Design review of the part built by this model. Coordinates are the model's own, in mm. Give positions to 0.01 mm unless a question says otherwise; leave off trailing zeros. Answer as a JSON object with one key per item and string values.
Autodesk Inventor part; units mm, degrees
ref_plane "Start Plane" through (0, 0, 0) normal (0, 0, 1) x (1, 0, 0)
ref_plane "End Plane" through (0, 0, 400) normal (0, 0, 1) x (1, 0, 0)
ref_plane "YZ Plane" through (0, 0, 0) normal (1, 0, 0) x (0, 1, 0)
ref_plane "Start Plane" through (0, 0, 0) normal (0, 0, 1) x (1, 0, 0)
ref_plane "End Plane" through (0, 0, 400) normal (0, 0, 1) x (1, 0, 0)
sketch "Sketch1" plane through (0, 0, 0) normal (0, 0, 1) x (1, 0, 0)
  line L0 (10, -4.5951) -> (10, -8.2)
  line L1 (-10, -8.2) -> (-10, -4.5951)
  line L2 (-10, 10) -> (10, -10) construction
  line L3 (10, 10) -> (-10, -10) construction
  circle A0 centre (0, 0) radius 2.1
  line L4 (-2.84, -3.9007) -> (2.84, -3.9007)
  line L5 (3.9007, -2.84) -> (3.9007, 2.84)
  line L6 (2.84, 3.9007) -> (-2.84, 3.9007)
  line L7 (-3.9007, 2.84) -> (-3.9007, -2.84)
  line L8 (-3.9007, -3.9007) -> (3.9007, 3.9007) construction
  line L9 (3.9007, -3.9007) -> (-3.9007, 3.9007) construction
  line L10 (-3.9007, -2.84) -> (-2.84, -3.9007) construction
  line L11 (-2.84, -3.9007) -> (-5.4993, -6.56)
  line L12 (-5.4993, -6.56) -> (-5.4993, -8.2)
  line L13 (-5.4993, -8.2) -> (-2.7951, -8.2)
  line L14 (-2.7951, -8.2) -> (-4.5951, -10)
  line L15 (0, 0) -> (0, -3.9007) construction
  line L16 (3.9007, -2.84) -> (2.84, -3.9007) construction
  line L17 (2.84, -3.9007) -> (5.4993, -6.56)
  line L18 (5.4993, -6.56) -> (5.4993, -8.2)
  line L19 (5.4993, -8.2) -> (2.7951, -8.2)
  line L20 (2.7951, -8.2) -> (4.5951, -10)
  line L21 (-2.84, -3.9007) -> (-3.9007, -2.84) construction
  line L22 (-3.9007, -2.84) -> (-6.56, -5.4993)
  line L23 (-6.56, -5.4993) -> (-8.2, -5.4993)
  line L24 (-8.2, -5.4993) -> (-8.2, -2.7951)
  line L25 (-8.2, -2.7951) -> (-10, -4.5951)
  line L26 (3.9007, -2.84) -> (6.56, -5.4993)
  line L27 (6.56, -5.4993) -> (8.2, -5.4993)
  line L28 (8.2, -5.4993) -> (8.2, -2.7951)
  line L29 (8.2, -2.7951) -> (10, -4.5951)
  arc A1 (-10, -8.2) -> (-8.2, -10) centre (-8.2, -8.2) ccw
  arc A2 (8.2, -10) -> (10, -8.2) centre (8.2, -8.2) ccw
  line L30 (-8.2, -6.56) -> (-7.7111, -6.56)
  line L31 (-6.6505, -8.2) -> (-8.2, -8.2)
  line L32 (-8.2, -8.2) -> (-8.2, -6.56)
  line L33 (-6.6505, -7.6207) -> (-7.7111, -6.56)
  line L34 (-6.6505, -7.6207) -> (-6.6505, -8.2)
  line L35 (8.2, -6.56) -> (7.7111, -6.56)
  line L36 (6.6505, -8.2) -> (8.2, -8.2)
  line L37 (8.2, -8.2) -> (8.2, -6.56)
  line L38 (6.6505, -7.6207) -> (7.7111, -6.56)
  line L39 (6.6505, -7.6207) -> (6.6505, -8.2)
  line L40 (8.2, -10) -> (4.5951, -10)
  line L41 (-4.5951, -10) -> (-8.2, -10)
  line L42 (-3.9007, 0) -> (3.9007, 0) construction
  line L43 (10, 4.5951) -> (10, 8.2)
  line L44 (-10, 8.2) -> (-10, 4.5951)
  line L45 (-2.84, 3.9007) -> (2.84, 3.9007)
  line L46 (-3.9007, 2.84) -> (-2.84, 3.9007) construction
  line L47 (-2.84, 3.9007) -> (-5.4993, 6.56)
  line L48 (-5.4993, 6.56) -> (-5.4993, 8.2)
  line L49 (-5.4993, 8.2) -> (-2.7951, 8.2)
  line L50 (-2.7951, 8.2) -> (-4.5951, 10)
  line L51 (2.84, 3.9007) -> (5.4993, 6.56)
  line L52 (5.4993, 6.56) -> (5.4993, 8.2)
  line L53 (5.4993, 8.2) -> (2.7951, 8.2)
  line L54 (2.7951, 8.2) -> (4.5951, 10)
  line L55 (3.9007, 2.84) -> (2.84, 3.9007) construction
  line L56 (-8.2, 2.7951) -> (-10, 4.5951)
  line L57 (-2.84, 3.9007) -> (-3.9007, 2.84) construction
  line L58 (-3.9007, 2.84) -> (-6.56, 5.4993)
  line L59 (-6.56, 5.4993) -> (-8.2, 5.4993)
  line L60 (-8.2, 5.4993) -> (-8.2, 2.7951)
  line L61 (3.9007, 2.84) -> (6.56, 5.4993)
  line L62 (6.56, 5.4993) -> (8.2, 5.4993)
  line L63 (8.2, 5.4993) -> (8.2, 2.7951)
  line L64 (8.2, 2.7951) -> (10, 4.5951)
  arc A3 (-8.2, 10) -> (-10, 8.2) centre (-8.2, 8.2) ccw
  arc A4 (10, 8.2) -> (8.2, 10) centre (8.2, 8.2) ccw
  line L65 (-8.2, 6.56) -> (-7.7111, 6.56)
  line L66 (-6.6505, 8.2) -> (-8.2, 8.2)
  line L67 (-8.2, 8.2) -> (-8.2, 6.56)
  line L68 (-6.6505, 7.6207) -> (-7.7111, 6.56)
  line L69 (-6.6505, 7.6207) -> (-6.6505, 8.2)
  line L70 (8.2, 6.56) -> (7.7111, 6.56)
  line L71 (6.6505, 7.6207) -> (7.7111, 6.56)
  line L72 (8.2, 8.2) -> (8.2, 6.56)
  line L73 (6.6505, 7.6207) -> (6.6505, 8.2)
  line L74 (6.6505, 8.2) -> (8.2, 8.2)
  line L75 (8.2, 10) -> (4.5951, 10)
  line L76 (-4.5951, 10) -> (-8.2, 10)
  line L77 (-8.2, 10) -> (-4.5951, 10)
  line L78 (4.5951, 10) -> (8.2, 10)
  point P0 (8.2, -8.2)
  point P1 (0, 3.9007)
  point P2 (8.2, 8.2)
  dimension "Width" = 20
  dimension "Height" = 20
  dimension "d2" = 4.2
  dimension "d3" = 1.5
  dimension "d4" = 1.64
  dimension "d6" = 5.68
  dimension "d7" = 1.8
  dimension "d9" = 1.5
extrude "Body" add sketch "Sketch1" along normal up to surface (400 mm away) from surface at 0
sketch "Sketch4" plane through (0, 0, 0) normal (0, 0, 1) x (1, 0, 0)
  line L0 (0, 0) -> (10, 0)
ref_plane "Work Plane4" through (0, 0, 0) normal (0, -1, 0) x (1, 0, 0)
sketch "Sketch5" plane through (0, 0, 0) normal (0, -1, 0) x (1, 0, 0)
  line L0 (-2, 0) -> (12, 0) construction
  line L1 (-2, 400) -> (12, 400) construction
  dimension "d17" = 400
equation "\"G_OFFSET_START\" = 0"
equation "\"G_OFFSET_END\" = 0"
equation "\"G_L\" = d17"
properties part number "400 mm V-Slot 20mm x 20mm" material "Aluminum 6061"
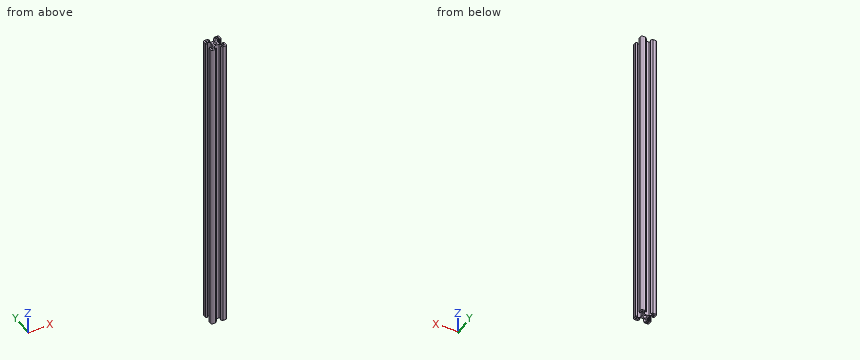
(1) To check wall thickness, follow L1, parallel to X at y = -8, z = 254.5; L2, parallel to Y at x = -8, z = 32.5; L3, parallel to Y at x = 0, z = 186.5. State the ranges of each line that lie inside material, in increasing order. Write a range as from..to.
Checked values:
{"L1": "x = -10..-8.2, -6.65..-5.5, 5.5..6.65, 8.2..10", "L2": "y = -10..-8.2, -6.56..-5.5, 5.5..6.56, 8.2..10", "L3": "y = -3.9..-2.1, 2.1..3.9"}
(2) Insertion check: pin 1 (5 mm diameter, centred on y = 1.5, z = 241, fed in from -X); pin 2 (1 mm diameter, centred on x = -4, z = 78.5, fed in from -Y); pin 3 (1.7 mm diameter, centred on x = 1, z = 137.5, fed in from +Y). Each pin has a flat end and moves straight along its axis. Give the tip position at first contact, or say it passes through.
Checked values:
{"pin 1": "stops at x = -9.4", "pin 2": "stops at y = -9.9", "pin 3": "stops at y = 3.9"}
(3) We need section A-A (z = 349.5). Count the separate pieces of the cut face and the enclosed holes in it, plus the area to 3 significant figures.
Checked values:
{"separate pieces": "1", "enclosed holes": "5", "area": "161 mm^2"}
